```python
from build123d import *
from OCP.BRepFilletAPI import BRepFilletAPI_MakeChamfer

# Parameters (mm, degrees)
SKETCH1_R           = 3.5
BOSS_EXTRUDE1_DEPTH = 18
SKETCH2_W           = 9
SKETCH2_H           = 2
BOSS_EXTRUDE3_DEPTH = 10
CUT_EXTRUDE3_START  = -8
SKETCH3_W           = 10
SKETCH3_H           = 4.5
CUT_EXTRUDE3_DEPTH  = 4
CHAMFER1_SIZE       = 1
CHAMFER1_SIZE2      = 0.577350269


with BuildPart() as part:
    # Sketch1 → Boss-Extrude1 (new body)
    with BuildSketch(Plane(origin=(0, 0, 0), x_dir=(1, 0, 0), z_dir=(0, 1, 0))):
        with Locations(Location((0, 0, 0), (0, 0, 270))):
            Circle(SKETCH1_R)
    extrude(amount=BOSS_EXTRUDE1_DEPTH)

    # Sketch2 → Boss-Extrude3 (add)
    with BuildSketch(Plane(origin=(0, 18, 0), x_dir=(1, 0, 0), z_dir=(0, 1, 0))):
        Rectangle(SKETCH2_W, SKETCH2_H)
    extrude(amount=-BOSS_EXTRUDE3_DEPTH)

    # Sketch3 → Cut-Extrude3 (cut)
    with BuildSketch(Plane.XZ.offset(CUT_EXTRUDE3_START)):
        with Locations((0, -1.25)):
            Rectangle(SKETCH3_W, SKETCH3_H)
    extrude(amount=-CUT_EXTRUDE3_DEPTH, mode=Mode.SUBTRACT)

    # Chamfer1: one chamfer whose edges measure the first distance from different faces: ONE call of the kernel's chamfer builder (chamfer() names one face for all edges)
    chamfer1_edges_1 = [part.edges().sort_by_distance(p)[0] for p in [
        (3.927050983, 18, -1),
    ]]
    chamfer1_side_1 = [part.faces().sort_by_distance(p)[0] for p in [
        (3.927050983, 15, -1),
    ]]
    chamfer1_edges_2 = [part.edges().sort_by_distance(p)[0] for p in [
        (3.927050983, 18, 1),
    ]]
    chamfer1_side_2 = [part.faces().sort_by_distance(p)[0] for p in [
        (3.927050983, 15, 1),
    ]]
    chamfer1_edges_3 = [part.edges().sort_by_distance(p)[0] for p in [
        (4.5, 18, 0),
    ]]
    chamfer1_side_3 = [part.faces().sort_by_distance(p)[0] for p in [
        (4.5, 15, 0),
    ]]
    chamfer1_edges_4 = [part.edges().sort_by_distance(p)[0] for p in [
        (-3.927050983, 18, 1),
    ]]
    chamfer1_side_4 = [part.faces().sort_by_distance(p)[0] for p in [
        (-3.927050983, 15, 1),
    ]]
    chamfer1_edges_5 = [part.edges().sort_by_distance(p)[0] for p in [
        (-3.927050983, 18, -1),
    ]]
    chamfer1_side_5 = [part.faces().sort_by_distance(p)[0] for p in [
        (-3.927050983, 15, -1),
    ]]
    chamfer1_edges_6 = [part.edges().sort_by_distance(p)[0] for p in [
        (-4.5, 18, 0),
    ]]
    chamfer1_side_6 = [part.faces().sort_by_distance(p)[0] for p in [
        (-4.5, 15, 0),
    ]]
    chamfer1_edges_7 = [part.edges().sort_by_distance(p)[0] for p in [
        (0, 18, -3.5),
    ]]
    chamfer1_side_7 = [part.faces().sort_by_distance(p)[0] for p in [
        (0, 15, -3.5),
    ]]
    chamfer1_edges_8 = [part.edges().sort_by_distance(p)[0] for p in [
        (2.091650066, 18, 2.80624304),
    ]]
    chamfer1_side_8 = [part.faces().sort_by_distance(p)[0] for p in [
        (0, 9, -3.5),
    ]]
    chamfer1 = BRepFilletAPI_MakeChamfer(part.part.solid().wrapped)
    for e in chamfer1_edges_1:
        chamfer1.Add(CHAMFER1_SIZE, CHAMFER1_SIZE2, e.wrapped, chamfer1_side_1[0].wrapped)  # the first distance lies on this face
    for e in chamfer1_edges_2:
        chamfer1.Add(CHAMFER1_SIZE, CHAMFER1_SIZE2, e.wrapped, chamfer1_side_2[0].wrapped)  # the first distance lies on this face
    for e in chamfer1_edges_3:
        chamfer1.Add(CHAMFER1_SIZE, CHAMFER1_SIZE2, e.wrapped, chamfer1_side_3[0].wrapped)  # the first distance lies on this face
    for e in chamfer1_edges_4:
        chamfer1.Add(CHAMFER1_SIZE, CHAMFER1_SIZE2, e.wrapped, chamfer1_side_4[0].wrapped)  # the first distance lies on this face
    for e in chamfer1_edges_5:
        chamfer1.Add(CHAMFER1_SIZE, CHAMFER1_SIZE2, e.wrapped, chamfer1_side_5[0].wrapped)  # the first distance lies on this face
    for e in chamfer1_edges_6:
        chamfer1.Add(CHAMFER1_SIZE, CHAMFER1_SIZE2, e.wrapped, chamfer1_side_6[0].wrapped)  # the first distance lies on this face
    for e in chamfer1_edges_7:
        chamfer1.Add(CHAMFER1_SIZE, CHAMFER1_SIZE2, e.wrapped, chamfer1_side_7[0].wrapped)  # the first distance lies on this face
    for e in chamfer1_edges_8:
        chamfer1.Add(CHAMFER1_SIZE, CHAMFER1_SIZE2, e.wrapped, chamfer1_side_8[0].wrapped)  # the first distance lies on this face
    add(Compound.cast(chamfer1.Shape()), mode=Mode.REPLACE)


solid = part.part
```
Read the model definition and answer for the solid it produces. Units are mm, in the model's axes. A direction names the side the tool comes from. Coordinates: 2 decimals unless noted, no trailing zeros. Loops run counter-clockwise (first coordinate to the right, second up) from the corner with the lowest first, then second, coordinate; pieces in that order, holes last. Notation, with made-up numbers: (5.25, 51) -> (32.25, 51) arc R12 cw to (32.25, 59) -> close; hole circle Ø10 at (66, 67.25). An arc over 180 degrees is marked (long way). Return JSON: item names as keys, results as strings.
Item 1: Find section B-B (y = 15.25). Determine the outline of the cut face in (x, z).
Answers:
{"outline": "(-4.5, -1) -> (-3.35, -1) arc R3.5 ccw to (3.35, -1) -> (4.5, -1) -> (4.5, 1) -> (3.35, 1) arc R3.5 ccw to (-3.35, 1) -> (-4.5, 1) -> close"}
Item 2: Flat-ended cylindrical pins translate along their axes: P1, Ø4, axis at x = -3, z = 1, coming from the -Y side; P2, Ø0.6, axis at x = 4, y = 13.5, coming from the +Z side; P3, Ø1.3, axis at x = -3.5, y = 13.5, coming from the +Z side. Find the tip coordinate at first contact, or state that the pin passes through.
Answers:
{"P1": "stops at y = 0", "P2": "stops at z = 1", "P3": "stops at z = 2.03"}
Item 3: Find section A-A (z = 0). Determine the outline of the cut face in (x, y).
Answers:
{"outline": "(-4.5, 12) -> (4.5, 12) -> (4.5, 17) -> (3.92, 18) -> (-3.92, 18) -> (-4.5, 17) -> close; (-3.5, 0) -> (3.5, 0) -> (3.5, 8) -> (-3.5, 8) -> close"}
Item 4: Find the intervals of material crossed by probe 1 along Y at (x, z) = (3, -0.25); probe 2 along X at (y, z) = (2.75, 0.5); probe 3 along X at (y, z) = (12.75, 1.25), in increasing order.
Answers:
{"probe 1": "y = 0 to 8, 12 to 18", "probe 2": "x = -3.46 to 3.46", "probe 3": "x = -3.27 to 3.27"}
Item 5: For faces 1 (the flat face through (-4, 15, -1)), 2 (the flat face through (-4, 15, 1)), 3 (the flat face through (4, 15, 1)), determine the directions among +Z, -Z, +X, -X, +Y, -Y from which every point of the face is accessible in a straight line to the end or side of a thin tool.
Answers:
{"face 1": "-Z, -X, +Y, -Y", "face 2": "+Z, -X, +Y, -Y", "face 3": "+Z, +X, +Y, -Y"}
Item 6: For a pull along Y with two mould halves and no side action, classify faces 4 (the flat face through (0, 18, 0)), 5 (the cylindrical face through (1.05, 6.49, 3.34)), 6 (the flat face through (0, 8, -1)) as +Y half, -Y half, draft (parallel to the pull), parting line (faces both ways), or undercut.
Answers:
{"face 4": "+Y half", "face 5": "draft", "face 6": "undercut"}
Item 7: Find section C-C (x = 0). Determine the outline of the cut face in (y, z), plus the area to 3 significant figures.
Answers:
{"outline": "(0, -3.5) -> (8, -3.5) -> (8, 1) -> (12, 1) -> (12, -3.5) -> (17, -3.5) -> (18, -2.92) -> (18, 2.92) -> (17, 3.5) -> (0, 3.5) -> close", "area": "107 mm2"}
Item 8: Find section D-D (y = 1.5). Determine the outline of the cut face in (x, z).
Answers:
{"outline": "circle Ø7 at (0, 0)"}
